Source: CAD feature listing. Evaluate the final solid. Frame: model axes, mm. A direction names the side the tool comes from. Coordinates: 2 decimals unless noted, no trailing zeros. Order: outer loops, then holes, each group sorted by start corner. A loop starts at its lowest first (then second) coordinate and runs counter-clockwise, first axis right, second up.
```python
from build123d import *

# Parameters (mm, degrees)
SKETCH2_R          = 5.77
CUT_EXTRUDE1_DEPTH = 1.87
SKETCH3_R          = 5.785
CUT_EXTRUDE2_DEPTH = 9.2
SKETCH4_R          = 5.675
CUT_EXTRUDE3_DEPTH = 54.6


with BuildPart() as part:
    # Sketch1 → Revolve1 (revolve)
    with BuildSketch(Plane.XY):
        Polygon((0, 20.722884615), (0, -44.947115385), (-6.845, -44.947115385), (-6.845, 9.652884615), (-7.095, 9.652884615), (-7.095, 18.852884615), (-13.675, 18.852884615), (-13.675, 20.722884615), align=None)
    revolve(axis=Axis((0, 20.722884615, 0), (0, -1, 0)))

    # Sketch2 → Cut-Extrude1 (cut)
    with BuildSketch(Plane(origin=(0, 20.722884615, 0), x_dir=(1, 0, 0), z_dir=(0, 1, 0))):
        Circle(SKETCH2_R)
    extrude(amount=-CUT_EXTRUDE1_DEPTH, mode=Mode.SUBTRACT)

    # Sketch3 → Cut-Extrude2 (cut)
    with BuildSketch(Plane(origin=(0, 18.852884615, 0), x_dir=(1, 0, 0), z_dir=(0, 1, 0))):
        Circle(SKETCH3_R)
    extrude(amount=-CUT_EXTRUDE2_DEPTH, mode=Mode.SUBTRACT)

    # Sketch4 → Cut-Extrude3 (cut)
    with BuildSketch(Plane(origin=(0, 9.652884615, 0), x_dir=(1, 0, 0), z_dir=(0, 1, 0))):
        Circle(SKETCH4_R)
    extrude(amount=-CUT_EXTRUDE3_DEPTH, mode=Mode.SUBTRACT)


solid = part.part
```
1. Access query for faces 1 (the face through (1.538, 14.317, 6.926)), 2 (the face through (5.242, -17.265, 2.174)). Directions: +Z, -Z, +X, -X, +Y, -Y. A direction counts if a zero-diameter tool reaches every point of the face in a straight line with its end or side. Return the directions, or none.
Findings:
face 1: -Y
face 2: +Y, -Y
2. Section query A-A on z = 0. Return loops of the section in (x, y) (3 decimals), plus the area to 3 significant figures.
Findings:
outline: (-13.675, 18.853) - (-7.095, 18.853) - (-7.095, 9.653) - (-6.845, 9.653) - (-6.845, -44.947) - (-5.675, -44.947) - (-5.675, 9.653) - (-5.785, 9.653) - (-5.785, 18.853) - (-5.77, 18.853) - (-5.77, 20.723) - (-13.675, 20.723) - close; (5.675, -44.947) - (6.845, -44.947) - (6.845, 9.653) - (7.095, 9.653) - (7.095, 18.853) - (13.675, 18.853) - (13.675, 20.723) - (5.77, 20.723) - (5.77, 18.853) - (5.785, 18.853) - (5.785, 9.653) - (5.675, 9.653) - close
area: 181 mm2
3. Draft query along X for faces 3 (the face through (-6, 20.723, 0)), 4 (the face through (5.504, 19.801, -1.733)), 5 (the face through (-7.4, 19.8, -11.5)). Return one class per face: released by +X, released by -X, zero draft, split by the parting line, or undercut.
Findings:
face 3: zero draft
face 4: undercut
face 5: split by the parting line
4. Pin query (flat end, axial travel): P1, Ø4, axis at x = 9.5, z = -6, coming from the -Y side; P2, Ø4, axis at x = 0.5, y = -38, coming from the -Z side (3 decimals); P3, Ø4, axis at y = -9.5, z = -6, coming from the -X side. Return the tip coordinate at first contact, or that it passes through.
Findings:
P1: stops at y = 18.85
P2: stops at z = -6.845
P3: stops at x = -5.55
5. Ray query, line 1 (Z direction, x = 0, y = 15.75) (3 decimals); line 2 (Z direction, x = 0, y = 19.3) (3 decimals); line 3 (X direction, y = -15, z = 0) (3 decimals). Return the intervals inside material, ascending.
Findings:
line 1: z = -7.095 to -5.785, 5.785 to 7.095
line 2: z = -13.675 to -5.77, 5.77 to 13.675
line 3: x = -6.845 to -5.675, 5.675 to 6.845
6. Section query D-D on x = -9. Return loops of the section in (y, z), plus the area to 3 significant figures.
Findings:
outline: (18.85, -10.3) - (20.72, -10.3) - (20.72, 10.3) - (18.85, 10.3) - close
area: 38.5 mm2
7. Section query C-C on y = 16. Return loops of the section in (x, z) (3 decimals).
Findings:
outline: circle Ø14.19 at (0, 0); hole circle Ø11.57 at (0, 0)
8. Section query B-B on x = 0. Return loops of the section in (y, z) (3 decimals).
Findings:
outline: (-44.947, -6.845) - (9.653, -6.845) - (9.653, -7.095) - (18.853, -7.095) - (18.853, -13.675) - (20.723, -13.675) - (20.723, -5.77) - (18.853, -5.77) - (18.853, -5.785) - (9.653, -5.785) - (9.653, -5.675) - (-44.947, -5.675) - close; (-44.947, 5.675) - (9.653, 5.675) - (9.653, 5.785) - (18.853, 5.785) - (18.853, 5.77) - (20.723, 5.77) - (20.723, 13.675) - (18.853, 13.675) - (18.853, 7.095) - (9.653, 7.095) - (9.653, 6.845) - (-44.947, 6.845) - close
